Geometry check sheet. Reference: the model listing, model coordinates, mm. A direction names the side the tool comes from. Give positions to 0.01 mm unless a question says otherwise; leave off trailing zeros. Loops run counter-clockwise (first coordinate to the right, second up) from the corner with the lowest first, then second, coordinate; pieces in that order, holes last. Notation, with made-up numbers: (85, -19.75) - (100, -19.75) arc R31 ccw to (100, 13.25) - close; hole circle Ø2 at (71, 80). An arc over 180 degrees is marked (long way). Use a Markdown table: item, result. Add a question column.
1. Material ranges on L1, parallel to X at y = 3.8, z = 63.5 (3 decimals); L2, parallel to X at y = 0.6, z = 68; L3, parallel to Z at x = -61, y = 2.85, recorded low to high.
2. Depth check by flat-ended pin: P1, Ø3, axis at x = -125, y = 2.5, coming from the -Z side; P2, Ø3, axis at y = 3.5, z = -91, coming from the +X side. Enter the tip coordinate at first touch or a pass-through.
3. Cross-section at C-C on x = -108. Enter the section's corners in (y, z), and give its area (3 significant figures).
4. Draft check along X on faces 1 (the flat face through (91.7, 3, 105)), 2 (the flat face through (-81, 3, -91.7)), 3 (the flat face through (115, 3, 69.7)). Enter one of: pulls with the +X half, pulls with the -X half, needs draft (parallel to the pull), parting line crosses it, or undercut.
5. Set-up check for faces 4 (the flat face through (-81, 3, 86.5)), 5 (the flat face through (139.7, 3, 1)): record each of +Z, -Z, +X, -X, +Y, -Y from which the full face is reachable in a straight line by a thin tool's end or side.
6. Cross-section at B-B on y = 1.05. Count the separate pieces of the cut face and the enclosed holes in it, and give its area (3 significant figures).
7. Cross-section at A-A on z = 63.5. Enter the section's corners in (x, y) (3 decimals).
from build123d import *

# Parameters (mm, degrees)
SKETCH1_W           = 279.4
SKETCH1_H           = 279.4
BOSS_EXTRUDE1_DEPTH = 5.9944
SKETCH2_W           = 48
SKETCH2_H           = 70
CUT_EXTRUDE1_DEPTH  = 198.656552715
SKETCH3_R           = 2.6
CUT_EXTRUDE2_DEPTH  = 198.656552715
FILLET1_R           = 2.54
SKETCH4_R           = 7.125
CUT_EXTRUDE3_DEPTH  = 198.656552715


with BuildPart() as part:
    # Sketch1 → Boss-Extrude1 (new body)
    with BuildSketch(Plane(origin=(0, 0, 0), x_dir=(1, 0, 0), z_dir=(0, 1, 0))):
        Rectangle(SKETCH1_W, SKETCH1_H)
    extrude(amount=BOSS_EXTRUDE1_DEPTH)

    # Sketch2 → Cut-Extrude1 (cut, through all)
    with BuildSketch(Plane(origin=(0, 5.9944, 0), x_dir=(1, 0, 0), z_dir=(0, 1, 0))):
        with Locations((-115.7, 104.7)):
            Rectangle(SKETCH2_W, SKETCH2_H)
        with Locations((115.7, 104.7)):
            Rectangle(SKETCH2_W, SKETCH2_H)
        with Locations((-115.7, -104.7)):
            Rectangle(SKETCH2_W, SKETCH2_H)
        with Locations((115.7, -104.7)):
            Rectangle(SKETCH2_W, SKETCH2_H)
    extrude(amount=-CUT_EXTRUDE1_DEPTH, mode=Mode.SUBTRACT)

    # Sketch3 → Cut-Extrude2 (cut, through all)
    with BuildSketch(Plane(origin=(0, 5.9944, 0), x_dir=(1, 0, 0), z_dir=(0, 1, 0))):
        with Locations(Location((-64.9, 120.3, 0), (0, 0, 270))):
            Circle(SKETCH3_R)
        with Locations(Location((-64.9, 89.1, 0), (0, 0, 270))):
            Circle(SKETCH3_R)
        with Locations(Location((64.9, 89.1, 0), (0, 0, 270))):
            Circle(SKETCH3_R)
        with Locations(Location((64.9, 120.3, 0), (0, 0, 270))):
            Circle(SKETCH3_R)
        with Locations(Location((64.9, -120.3, 0), (0, 0, 270))):
            Circle(SKETCH3_R)
        with Locations(Location((64.9, -89.1, 0), (0, 0, 270))):
            Circle(SKETCH3_R)
        with Locations(Location((-64.9, -89.1, 0), (0, 0, 270))):
            Circle(SKETCH3_R)
        with Locations(Location((-64.9, -120.3, 0), (0, 0, 270))):
            Circle(SKETCH3_R)
        with BuildLine():
            Line((-84.1, 122.9), (-77.7, 122.9))
            ThreePointArc((-77.7, 122.9), (-75.1, 120.3), (-77.7, 117.7))
            Line((-77.7, 117.7), (-84.1, 117.7))
            ThreePointArc((-84.1, 117.7), (-86.7, 120.3), (-84.1, 122.9))
        make_face()
        with BuildLine():
            Line((-52.1, 122.9), (-45.7, 122.9))
            ThreePointArc((-45.7, 122.9), (-43.1, 120.3), (-45.7, 117.7))
            Line((-45.7, 117.7), (-52.1, 117.7))
            ThreePointArc((-52.1, 117.7), (-54.7, 120.3), (-52.1, 122.9))
        make_face()
        with BuildLine():
            Line((-84.1, 91.7), (-77.7, 91.7))
            ThreePointArc((-77.7, 91.7), (-75.1, 89.1), (-77.7, 86.5))
            Line((-77.7, 86.5), (-84.1, 86.5))
            ThreePointArc((-84.1, 86.5), (-86.7, 89.1), (-84.1, 91.7))
        make_face()
        with BuildLine():
            Line((-52.1, 91.7), (-45.7, 91.7))
            ThreePointArc((-45.7, 91.7), (-43.1, 89.1), (-45.7, 86.5))
            Line((-45.7, 86.5), (-52.1, 86.5))
            ThreePointArc((-52.1, 86.5), (-54.7, 89.1), (-52.1, 91.7))
        make_face()
        with BuildLine():
            Line((52.1, 91.7), (45.7, 91.7))
            ThreePointArc((45.7, 91.7), (43.1, 89.1), (45.7, 86.5))
            Line((45.7, 86.5), (52.1, 86.5))
            ThreePointArc((52.1, 86.5), (54.7, 89.1), (52.1, 91.7))
        make_face()
        with BuildLine():
            Line((84.1, 91.7), (77.7, 91.7))
            ThreePointArc((77.7, 91.7), (75.1, 89.1), (77.7, 86.5))
            Line((77.7, 86.5), (84.1, 86.5))
            ThreePointArc((84.1, 86.5), (86.7, 89.1), (84.1, 91.7))
        make_face()
        with BuildLine():
            Line((52.1, 122.9), (45.7, 122.9))
            ThreePointArc((45.7, 122.9), (43.1, 120.3), (45.7, 117.7))
            Line((45.7, 117.7), (52.1, 117.7))
            ThreePointArc((52.1, 117.7), (54.7, 120.3), (52.1, 122.9))
        make_face()
        with BuildLine():
            Line((84.1, 122.9), (77.7, 122.9))
            ThreePointArc((77.7, 122.9), (75.1, 120.3), (77.7, 117.7))
            Line((77.7, 117.7), (84.1, 117.7))
            ThreePointArc((84.1, 117.7), (86.7, 120.3), (84.1, 122.9))
        make_face()
        with BuildLine():
            Line((-84.1, -122.9), (-77.7, -122.9))
            ThreePointArc((-77.7, -122.9), (-75.1, -120.3), (-77.7, -117.7))
            Line((-77.7, -117.7), (-84.1, -117.7))
            ThreePointArc((-84.1, -117.7), (-86.7, -120.3), (-84.1, -122.9))
        make_face()
        with BuildLine():
            Line((-52.1, -122.9), (-45.7, -122.9))
            ThreePointArc((-45.7, -122.9), (-43.1, -120.3), (-45.7, -117.7))
            Line((-45.7, -117.7), (-52.1, -117.7))
            ThreePointArc((-52.1, -117.7), (-54.7, -120.3), (-52.1, -122.9))
        make_face()
        with BuildLine():
            Line((-84.1, -91.7), (-77.7, -91.7))
            ThreePointArc((-77.7, -91.7), (-75.1, -89.1), (-77.7, -86.5))
            Line((-77.7, -86.5), (-84.1, -86.5))
            ThreePointArc((-84.1, -86.5), (-86.7, -89.1), (-84.1, -91.7))
        make_face()
        with BuildLine():
            Line((-52.1, -91.7), (-45.7, -91.7))
            ThreePointArc((-45.7, -91.7), (-43.1, -89.1), (-45.7, -86.5))
            Line((-45.7, -86.5), (-52.1, -86.5))
            ThreePointArc((-52.1, -86.5), (-54.7, -89.1), (-52.1, -91.7))
        make_face()
        with BuildLine():
            Line((52.1, -91.7), (45.7, -91.7))
            ThreePointArc((45.7, -91.7), (43.1, -89.1), (45.7, -86.5))
            Line((45.7, -86.5), (52.1, -86.5))
            ThreePointArc((52.1, -86.5), (54.7, -89.1), (52.1, -91.7))
        make_face()
        with BuildLine():
            Line((84.1, -91.7), (77.7, -91.7))
            ThreePointArc((77.7, -91.7), (75.1, -89.1), (77.7, -86.5))
            Line((77.7, -86.5), (84.1, -86.5))
            ThreePointArc((84.1, -86.5), (86.7, -89.1), (84.1, -91.7))
        make_face()
        with BuildLine():
            Line((52.1, -122.9), (45.7, -122.9))
            ThreePointArc((45.7, -122.9), (43.1, -120.3), (45.7, -117.7))
            Line((45.7, -117.7), (52.1, -117.7))
            ThreePointArc((52.1, -117.7), (54.7, -120.3), (52.1, -122.9))
        make_face()
        with BuildLine():
            Line((84.1, -122.9), (77.7, -122.9))
            ThreePointArc((77.7, -122.9), (75.1, -120.3), (77.7, -117.7))
            Line((77.7, -117.7), (84.1, -117.7))
            ThreePointArc((84.1, -117.7), (86.7, -120.3), (84.1, -122.9))
        make_face()
    extrude(amount=-CUT_EXTRUDE2_DEPTH, mode=Mode.SUBTRACT)

    # Fillet1
    fillet1_edges = [part.edges().sort_by_distance(p)[0] for p in [
        (139.7, 2.9972, -69.7),
        (91.7, 2.9972, -69.7),
        (91.7, 2.9972, -139.7),
        (-139.7, 2.9972, 69.7),
        (-91.7, 2.9972, 69.7),
        (-91.7, 2.9972, 139.7),
        (139.7, 2.9972, 69.7),
        (91.7, 2.9972, 139.7),
        (91.7, 2.9972, 69.7),
        (-139.7, 2.9972, -69.7),
        (-91.7, 2.9972, -139.7),
        (-91.7, 2.9972, -69.7),
    ]]
    fillet(fillet1_edges, radius=FILLET1_R)

    # Sketch4 → Cut-Extrude3 (cut, through all)
    with BuildSketch(Plane(origin=(0, 5.9944, 0), x_dir=(1, 0, 0), z_dir=(0, 1, 0))):
        with Locations(Location((-63.5, 63.5, 0), (0, 0, 270))):
            Circle(SKETCH4_R)
        with Locations(Location((-63.5, -63.5, 0), (0, 0, 270))):
            Circle(SKETCH4_R)
        with Locations(Location((63.5, 63.5, 0), (0, 0, 270))):
            Circle(SKETCH4_R)
        with Locations(Location((63.5, -63.5, 0), (0, 0, 270))):
            Circle(SKETCH4_R)
    extrude(amount=-CUT_EXTRUDE3_DEPTH, mode=Mode.SUBTRACT)


solid = part.part
Values found:
| question | item | result |
|---|---|---|
| 1 | L1 | x = -139.7 to -70.625, -56.375 to 56.375, 70.625 to 139.7 |
| 1 | L2 | x = -139.56 to -69.02, -57.98 to 57.98, 69.02 to 139.56 |
| 1 | L3 | z = -139.7 to -70.17, -56.83 to 56.83, 70.17 to 139.7 |
| 2 | P1 | stops at z = -69.7 |
| 2 | P2 | stops at x = 91.7 |
| 3 | outline | (0, -69.7) - (5.99, -69.7) - (5.99, 69.7) - (0, 69.7) - close |
| 3 | area | 836 mm2 |
| 4 | face 1 | pulls with the +X half |
| 4 | face 2 | undercut |
| 4 | face 3 | needs draft |
| 5 | face 4 | +Y, -Y |
| 5 | face 5 | +Z, -Z, +X, +Y, -Y |
| 6 | separate pieces | 1 |
| 6 | enclosed holes | 28 |
| 6 | area | 62,900 mm2 |
| 7 | outline | (-139.7, 0) - (-70.625, 0) - (-70.625, 5.994) - (-139.7, 5.994) - close; (-56.375, 0) - (56.375, 0) - (56.375, 5.994) - (-56.375, 5.994) - close; (70.625, 0) - (139.7, 0) - (139.7, 5.994) - (70.625, 5.994) - close |
